Input: dimensioned drawing with shaded views. Units: mm. Origin: part minimum x, y, z. A direction names the side the tool comes from. Coordinates: 2 decimals unless noted, no trailing zeros. Order: outer loops, then holes, each group sorted by start corner. A loop starts at its lowest first (then second) coordinate and runs counter-clockwise, first axis right, second up. Notation, with made-up numbers: (83.25, 78.5) -> (138.25, 78.5) arc R38 cw to (138.25, 116.5) -> close; hole circle Ø1 at (23, 23.25). An arc over 180 degrees is marked (long way). Answer in a Markdown table with one row per item. Add a question column.
1) Contact query for flat-ended pins moving along their axis: P1, Ø1.5, axis at x = 7.5, y = 5.5, coming from the +Z side (3 decimals); P2, Ø1.5, axis at x = 14, y = 11, coming from the +Z side. Output: stop coordinate, or through.
2) Section query A-A on z = 10. Return the cut outline in (x, y) (3 decimals), then the cut area to 3 significant figures.
3) Ray query, line 1 (X direction, y = 19.5, z = 14.5) (3 decimals); line 2 (Y direction, x = 25.5, z = 15.25). Return the intervals inside material, ascending. Write a range as from..to.
4) Section query B-B on x = 10.5. Return the cut outline in (y, z) (3 decimals).
5) Set-up query: the marked faces 1 and 2. Return all of +Z, -Z, +X, -X, +Y, -Y with unobstructed straight access to the full face (end or side cutting, diameter ignored); none if empty.
6) Pull-direction query (X, two-part tool) for the marked faces 3, 4 and 5; classes: +X half, -X half, draft (parallel to the pull), parting line (faces both ways), or undercut.
7) Section query C-C on y = 14. Return the cut outline in (x, z) (3 decimals).
8) Section query D-D on y = 4. Return the cut outline in (x, z) (3 decimals).
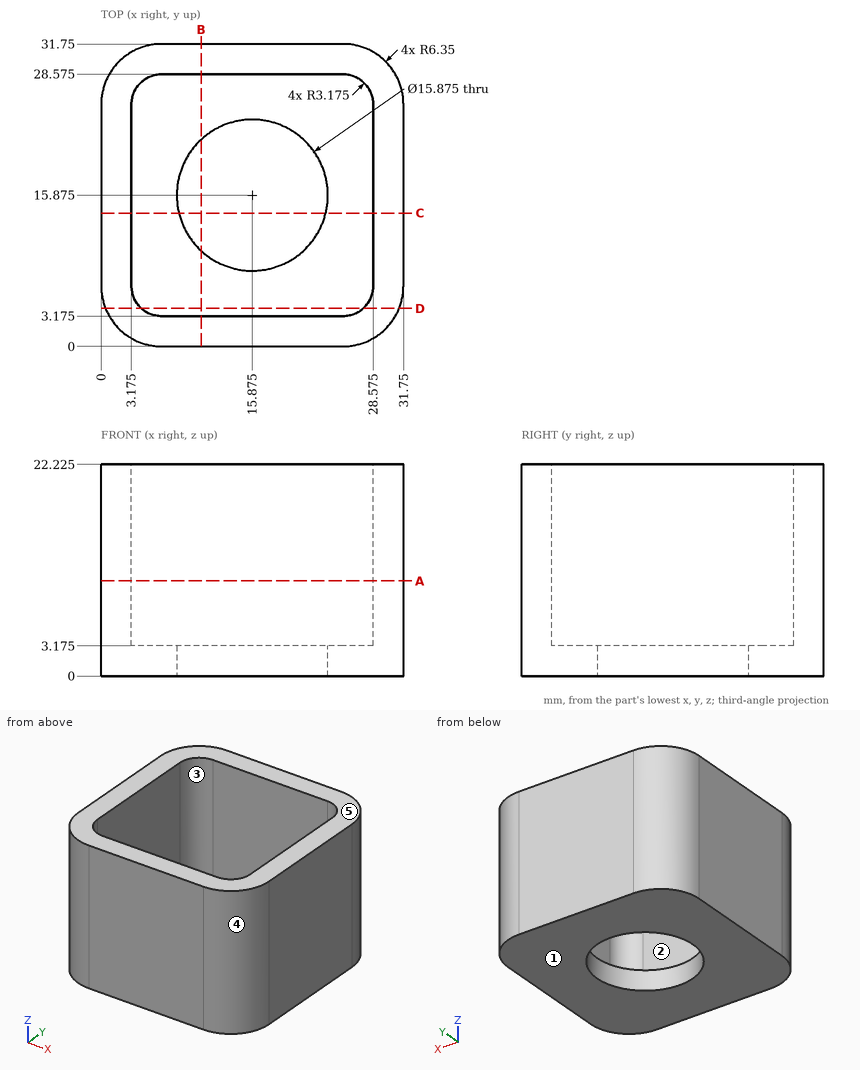
Result:
| question | item | result |
|---|---|---|
| 1 | P1 | z = 3.175 |
| 1 | P2 | through |
| 2 | outline | (0, 6.35) arc R6.35 ccw to (6.35, 0) -> (25.4, 0) arc R6.35 ccw to (31.75, 6.35) -> (31.75, 25.4) arc R6.35 ccw to (25.4, 31.75) -> (6.35, 31.75) arc R6.35 ccw to (0, 25.4) -> close; hole (3.175, 6.35) arc R3.175 ccw to (6.35, 3.175) -> (25.4, 3.175) arc R3.175 ccw to (28.575, 6.35) -> (28.575, 25.4) arc R3.175 ccw to (25.4, 28.575) -> (6.35, 28.575) arc R3.175 ccw to (3.175, 25.4) -> close |
| 2 | area | 337 mm2 |
| 3 | line 1 | 0..3.175, 28.575..31.75 |
| 3 | line 2 | 0..3.18, 28.57..31.75 |
| 4 | outline | (0, 0) -> (10.034, 0) -> (10.034, 3.175) -> (3.175, 3.175) -> (3.175, 22.225) -> (0, 22.225) -> close; (21.716, 0) -> (31.75, 0) -> (31.75, 22.225) -> (28.575, 22.225) -> (28.575, 3.175) -> (21.716, 3.175) -> close |
| 5 | face 1 | -Z, +X, -X, +Y, -Y |
| 5 | face 2 | +Z |
| 6 | face 3 | undercut |
| 6 | face 4 | +X half |
| 6 | face 5 | draft |
| 7 | outline | (0, 0) -> (8.162, 0) -> (8.162, 3.175) -> (3.175, 3.175) -> (3.175, 22.225) -> (0, 22.225) -> close; (23.588, 0) -> (31.75, 0) -> (31.75, 22.225) -> (28.575, 22.225) -> (28.575, 3.175) -> (23.588, 3.175) -> close |
| 8 | outline | (0.451, 0) -> (31.299, 0) -> (31.299, 22.225) -> (27.535, 22.225) -> (27.535, 3.175) -> (4.215, 3.175) -> (4.215, 22.225) -> (0.451, 22.225) -> close |
